```python
from build123d import *

# Parameters (mm, degrees)
SKETCH2_W           = 5.4034
SKETCH2_H           = 22.6066
SKETCH2_W_2         = 31.9679
SKETCH2_H_2         = 18.2371
BOSS_EXTRUDE1_DEPTH = 3.048
SKETCH3_R           = 1.338245378
CUT_EXTRUDE1_DEPTH  = 4.048
SKETCH4_R           = 1.524
CUT_EXTRUDE2_DEPTH  = 4.048


with BuildPart() as part:
    # Sketch2 → Boss-Extrude1 (new body)
    with BuildSketch(Plane(origin=(0, 0, 8.171752382), x_dir=(-1, 0, 0), z_dir=(0, 0, -1))):
        with BuildLine():
            Line((-23.844892625, -33.084405696), (-34.084892625, -36.451005696))
            ThreePointArc((-34.084892625, -36.451005696), (-36.778969461, -35.335082532), (-37.894892625, -32.641005696))
            Line((-37.894892625, -32.641005696), (-37.894892625, 26.697694304))
            ThreePointArc((-37.894892625, 26.697694304), (-36.778969461, 29.391771141), (-34.084892625, 30.507694304))
            Line((-34.084892625, 30.507694304), (57.404932375, 30.507694304))
            ThreePointArc((57.404932375, 30.507694304), (60.103884597, 29.386886916), (61.214907375, 26.683892153))
            Line((61.214907375, 26.683892153), (61.214907375, 24.068294304))
            Line((61.214907375, 24.068294304), (40.134807375, 24.068294304))
            Line((40.134807375, 24.068294304), (40.134807375, 8.658194304))
            Line((40.134807375, 8.658194304), (56.975007375, 8.658194304))
            Line((56.975007375, 8.658194304), (56.975007375, 4.997894304))
            Line((56.975007375, 4.997894304), (40.134807375, 4.997894304))
            Line((40.134807375, 4.997894304), (40.134807375, -9.121805696))
            Line((40.134807375, -9.121805696), (56.975007375, -9.121805696))
            Line((56.975007375, -9.121805696), (56.975007375, -12.628005696))
            Line((56.975007375, -12.628005696), (35.575007375, -12.628005696))
            Line((35.575007375, -12.628005696), (35.575007375, -28.627805696))
            Line((35.575007375, -28.627805696), (61.214907375, -28.627805696))
            Line((61.214907375, -28.627805696), (61.214907375, -32.613401529))
            ThreePointArc((61.214907375, -32.613401529), (60.108826144, -35.325305244), (57.405007375, -36.451005696))
            Line((57.405007375, -36.451005696), (38.714307375, -36.451005696))
            Line((38.714307375, -36.451005696), (28.474307375, -33.084405696))
            Line((28.474307375, -33.084405696), (28.474307375, -18.034905696))
            Line((28.474307375, -18.034905696), (20.658107375, -18.034905696))
            Line((20.658107375, -18.034905696), (20.658107375, -33.084405696))
            Line((20.658107375, -33.084405696), (10.926407375, -33.084405696))
            Line((10.926407375, -33.084405696), (10.926407375, -20.384405696))
            Line((10.926407375, -20.384405696), (-5.302892625, -20.384405696))
            Line((-5.302892625, -20.384405696), (-5.302892625, -33.084405696))
            Line((-5.302892625, -33.084405696), (-23.844892625, -33.084405696))
        make_face()
        with Locations((16.546707375, -19.663505696)):
            Rectangle(SKETCH2_W, SKETCH2_H, mode=Mode.SUBTRACT)
        Polygon((-29.004892625, -23.698905696), (-22.066892625, -23.698905696), (-22.066892625, -21.185805696), (-19.950892625, -21.185805696), (-19.950892625, -18.920605696), (-17.244692625, -18.920605696), (-17.244692625, -10.792605696), (-23.416892625, -10.792605696), (-23.416892625, 9.801194304), (-29.004892625, 9.801194304), align=None, mode=Mode.SUBTRACT)
        with Locations((-5.654942625, 1.475544304)):
            Rectangle(SKETCH2_W_2, SKETCH2_H_2, mode=Mode.SUBTRACT)
        Polygon((12.361007375, -0.097605696), (17.441007375, -0.097605696), (17.441007375, 15.972394304), (37.825007375, 15.972394304), (37.825007375, 8.658194304), (32.872007375, 8.658194304), (32.872007375, -5.431505696), (12.361007375, -5.431505696), align=None, mode=Mode.SUBTRACT)
        Polygon((0.677107375, 12.372094304), (-29.004794688, 12.372094304), (-29.004892625, 25.896994304), (31.688307375, 25.896994304), (31.688307375, 18.086994304), (0.677107375, 18.086994304), align=None, mode=Mode.SUBTRACT)
    extrude(amount=BOSS_EXTRUDE1_DEPTH)

    # Sketch3 → Cut-Extrude1 (cut, through all)
    with BuildSketch(Plane(origin=(0, 0, 5.123752382), x_dir=(-1, 0, 0), z_dir=(0, 0, -1))):
        with Locations((57.405007375, -32.641005696)):
            Circle(SKETCH3_R)
        with Locations((-34.084892625, -32.641005696)):
            Circle(SKETCH3_R)
        with Locations((-34.084892625, 26.697694304)):
            Circle(SKETCH3_R)
        with Locations((57.404932375, 26.697694304)):
            Circle(SKETCH3_R)
    extrude(amount=-CUT_EXTRUDE1_DEPTH, mode=Mode.SUBTRACT)

    # Sketch4 → Cut-Extrude2 (cut, through all)
    with BuildSketch(Plane(origin=(0, 0, 5.123752382), x_dir=(-1, 0, 0), z_dir=(0, 0, -1))):
        with Locations((-34.084892625, 26.697694304)):
            Circle(SKETCH4_R)
        with Locations((-34.084892625, -32.641005696)):
            Circle(SKETCH4_R)
        with Locations((57.405007375, -32.641005696)):
            Circle(SKETCH4_R)
        with Locations((57.404932375, 26.697694304)):
            Circle(SKETCH4_R)
    extrude(amount=-CUT_EXTRUDE2_DEPTH, mode=Mode.SUBTRACT)


solid = part.part
```
Input: part model. Units: mm. Frame: model coordinates. A direction names the side the tool comes from. Round coordinates to 2 decimals unless told otherwise and drop trailing zeros. Loops run counter-clockwise (first coordinate to the right, second up) from the corner with the lowest first, then second, coordinate; pieces in that order, holes last.
1) Pull-direction query (X, two-part tool) for faces 4 (the flat face through (-15, -0.098, 7)), 5 (the flat face through (-48, 8.658, 7)); classes: released by +X, released by -X, zero draft, split by the parting line, or undercut.
Ans:
face 4: undercut
face 5: zero draft
2) Material intervals for line 1 (X direction, y = -15, z = 7.35) (3 decimals); line 2 (X direction, y = -23, z = 8) (3 decimals); line 3 (X direction, y = 14, z = 6.25) (3 decimals), sorted ascending.
Ans:
line 1: x = -35.575 to -19.248, -13.845 to 17.245, 29.005 to 37.895
line 2: x = -35.575 to -28.474, -20.658 to -19.248, -13.845 to -10.926, 5.303 to 22.067, 29.005 to 37.895
line 3: x = -40.135 to -37.825, -17.441 to -0.677, 29.005 to 37.895
3) Pin query (flat end, axial travel): pin 1 (1.5 mm diameter, centred on y = -22, z = 6.5, fed in from -X) (3 decimals); pin 2 (1.5 mm diameter, centred on x = -24, z = 7.5, fed in from -Y). Return the tip coordinate at first contact, or that it passes through.
Ans:
pin 1: stops at x = -35.575
pin 2: stops at y = -18.03
4) Set-up query: faces 1 (the flat face through (-28.474, -26, 7)), 2 (the flat face through (-1, -10, 5.124)), 3 (the flat face through (-17, -30.967, 7)). Return all of +Z, -Z, +X, -X, +Y, -Y with unobstructed straight access to the full face (end or side cutting, diameter ignored); none if empty.
Ans:
face 1: +Z, -Z, -Y
face 2: -Z, +X, -X, +Y, -Y
face 3: +Z, -Z
5) Section query B-B on y = -25. Return the cut outline in (x, z) (3 decimals), plus the area to 3 significant figures.
Ans:
outline: (-35.575, 5.124) - (-28.474, 5.124) - (-28.474, 8.172) - (-35.575, 8.172) - close; (-20.658, 5.124) - (-19.248, 5.124) - (-19.248, 8.172) - (-20.658, 8.172) - close; (-13.845, 5.124) - (-10.926, 5.124) - (-10.926, 8.172) - (-13.845, 8.172) - close; (5.303, 5.124) - (37.895, 5.124) - (37.895, 8.172) - (5.303, 8.172) - close
area: 134 mm2
6) Section query C-C on y = 21. Return the cut outline in (x, z).
Ans:
outline: (-40.13, 5.12) - (-31.69, 5.12) - (-31.69, 8.17) - (-40.13, 8.17) - close; (29, 5.12) - (37.89, 5.12) - (37.89, 8.17) - (29, 8.17) - close
7) Section query D-D on z = 6.3. Count the separate pieces of the cut face and the enclosed holes in it, plus the area to 3 significant figures.
Ans:
separate pieces: 1
enclosed holes: 9
area: 3,010 mm2
8) Section query A-A on x = -4. Return the cut outline in (y, z), plus the area to 3 significant figures.
Ans:
outline: (-20.38, 5.12) - (-7.64, 5.12) - (-7.64, 8.17) - (-20.38, 8.17) - close; (10.59, 5.12) - (18.09, 5.12) - (18.09, 8.17) - (10.59, 8.17) - close; (25.9, 5.12) - (30.51, 5.12) - (30.51, 8.17) - (25.9, 8.17) - close
area: 75.7 mm2
